Geometry: final body of the model. Coordinates: model frame, mm. Face numbers are marked on the shaded views. A direction names the side the tool comes from. Give positions to 0.01 mm unless a question says otherwise; leave off trailing zeros. Write each loop counter-clockwise with the first axis right and the second up, starting at its lowest first coordinate (ties: lowest second). Pieces come first, ordered by that corner, then holes. Notation, with made-up numbers: (12.5, 57) -> (45.5, 57) arc R15 ccw to (45.5, 67) -> close; hole circle Ø1 at (82.25, 73). An arc over 180 degrees is marked (long way). Answer as a JSON object with one key per item and string values.
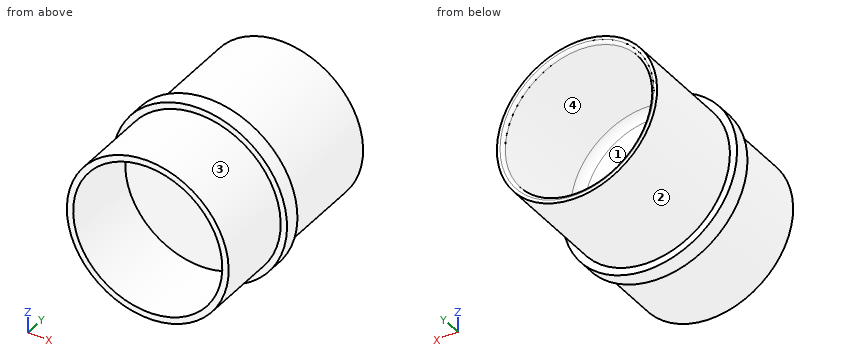
from build123d import *

# Parameters (mm, degrees)
SKETCH1_R           = 25.5
SKETCH1_R_2         = 23.5
BOSS_EXTRUDE1_DEPTH = 25
SKETCH2_R           = 27.5
BOSS_EXTRUDE2_DEPTH = 5
SKETCH3_R           = 25.25
SKETCH3_R_2         = 23.25
BOSS_EXTRUDE3_DEPTH = 35
FILLET1_R           = 2.54
FILLET2_R           = 1


with BuildPart() as part:
    # Sketch1 → Boss-Extrude1 (new body)
    with BuildSketch(Plane(origin=(0, 0, 0), x_dir=(1, 0, 0), z_dir=(0, 1, 0))):
        with Locations(Location((0, 0, 0), (0, 0, 270))):
            Circle(SKETCH1_R)
        with Locations(Location((0, 0, 0), (0, 0, 270))):
            Circle(SKETCH1_R_2, mode=Mode.SUBTRACT)
    extrude(amount=BOSS_EXTRUDE1_DEPTH)

    # Sketch2 → Boss-Extrude2 (add)
    with BuildSketch(Plane(origin=(0, 25, 0), x_dir=(1, 0, 0), z_dir=(0, 1, 0))):
        with Locations(Location((0, 0, 0), (0, 0, 270))):
            Circle(SKETCH2_R)
    extrude(amount=BOSS_EXTRUDE2_DEPTH)

    # Sketch3 → Boss-Extrude3 (add)
    with BuildSketch(Plane(origin=(0, 30, 0), x_dir=(1, 0, 0), z_dir=(0, 1, 0))):
        with Locations(Location((0, 0, 0), (0, 0, 270))):
            Circle(SKETCH3_R)
        with Locations(Location((0, 0, 0), (0, 0, 270))):
            Circle(SKETCH3_R_2, mode=Mode.SUBTRACT)
    extrude(amount=BOSS_EXTRUDE3_DEPTH)

    # Fillet1
    fillet1_edges = [part.edges().sort_by_distance(p)[0] for p in [
        (0, 30, -23.25),
    ]]
    fillet(fillet1_edges, radius=FILLET1_R)

    # Fillet2
    fillet2_edges = [part.edges().sort_by_distance(p)[0] for p in [
        (0, 65, -23.25),
    ]]
    fillet(fillet2_edges, radius=FILLET2_R)


solid = part.part
Q1. Mould query, pull axis X, two halves, no side actions, for the marked faces 1 and 2. Classes: pulls with the +X half, pulls with the -X half, needs draft (parallel to the pull), parting line crosses it, or undercut.
Values:
{"face 1": "undercut", "face 2": "parting line crosses it"}
Q2. Cut plane C-C (y = 8). Return the cut outline in (x, z), and give its area (3 significant figures).
Values:
{"outline": "circle Ø51 at (0, 0); hole circle Ø47 at (0, 0)", "area": "308 mm²"}
Q3. Cut plane A-A (x = 0). Return the cut outline in (y, z), and give its area (3 significant figures).
Values:
{"outline": "(0, -25.5) -> (25, -25.5) -> (25, -27.5) -> (30, -27.5) -> (30, -25.25) -> (65, -25.25) -> (65, -24.25) arc R1 ccw to (64, -23.25) -> (32.54, -23.25) arc R2.54 cw to (30, -20.71) -> (30, 20.71) arc R2.54 cw to (32.54, 23.25) -> (64, 23.25) arc R1 ccw to (65, 24.25) -> (65, 25.25) -> (30, 25.25) -> (30, 27.5) -> (25, 27.5) -> (25, 25.5) -> (0, 25.5) -> (0, 23.5) -> (25, 23.5) -> (25, -23.5) -> (0, -23.5) -> close", "area": "517 mm²"}
Q4. Material intervals for L1, parallel to X at y = 51, z = 0; L2, parallel to X at y = 7, z = 0; L3, parallel to Y at x = -17, z = 20, sorted ascending. Write a range as from..to.
Values:
{"L1": "-25.25..-23.25, 23.25..25.25", "L2": "-25.5..-23.5, 23.5..25.5", "L3": "25..30"}
Q5. Set-up query: the marked faces 3 and 4. Return all of +Z, -Z, +X, -X, +Y, -Y with unobstructed straight access to the full face (end or side cutting, diameter ignored); none if empty.
Values:
{"face 3": "-Y", "face 4": "+Y"}
Q6. First-contact query: P1, Ø16.5, axis at x = 2, z = -13, coming from the +Y side; P2, Ø4, axis at x = -3.5, z = -1, coming from the -Y side; P3, Ø2, axis at x = -10, y = 47.5, coming from the +Z side; P4, Ø10, axis at x = -2, z = -19.5, coming from the -Y side. Flat tips, straight axial feed; report the tip coordinate or a pass-through.
Values:
{"P1": "y = 30.1", "P2": "y = 25", "P3": "z = 23.59", "P4": "y = 0"}
Q7. Cut plane B-B (z = 0). Return the cut outline in (x, y).
Values:
{"outline": "(-27.5, 25) -> (-25.5, 25) -> (-25.5, 0) -> (-23.5, 0) -> (-23.5, 25) -> (23.5, 25) -> (23.5, 0) -> (25.5, 0) -> (25.5, 25) -> (27.5, 25) -> (27.5, 30) -> (25.25, 30) -> (25.25, 65) -> (24.25, 65) arc R1 ccw to (23.25, 64) -> (23.25, 32.54) arc R2.54 cw to (20.71, 30) -> (-20.71, 30) arc R2.54 cw to (-23.25, 32.54) -> (-23.25, 64) arc R1 ccw to (-24.25, 65) -> (-25.25, 65) -> (-25.25, 30) -> (-27.5, 30) -> close"}
Q8. Cut plane D-D (y = 28). Return the cut outline in (x, z).
Values:
{"outline": "circle Ø55 at (0, 0)"}
